```python
from build123d import *

# Parameters (mm, degrees)
FURO_COM_FOLGA_DE_M61_D = 6.4


with BuildPart() as part:
    # Esbo_o1 → Revolu_o1 (revolve)
    with BuildSketch(Plane(origin=(0, 0, 0), x_dir=(0, 0, -1), z_dir=(1, 0, 0)), mode=Mode.PRIVATE) as revolu_o1_sk:
        Polygon((-2, 6.5), (0, 6.5), (0, 0), (-7, 0), (-7, 6.5), (-4.7, 6.5), (-4.7, 4.3), (-2, 4.3), align=None)
    revolve(revolu_o1_sk.sketch.rotate(Axis((0, 0, 7), (0, 0, -1)), 90), axis=Axis((0, 0, 7), (0, 0, -1)))

    # Furo com folga de M61 (through all)
    with Locations(Plane(origin=(0, 0, 0), x_dir=(-1, 0, 0), z_dir=(0, 0, -1))):
        with Locations((0, 0)):
            Hole(FURO_COM_FOLGA_DE_M61_D / 2)


solid = part.part
```
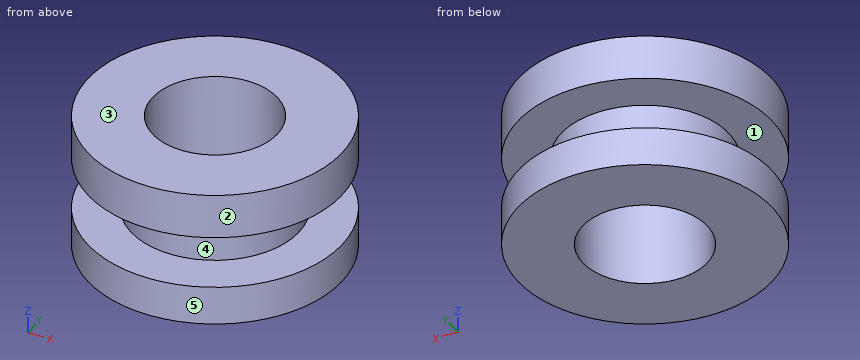
Input: part model. Units: mm. Frame: model coordinates. Face numbers are marked on the shaded views. A direction names the side the tool comes from. Round coordinates to 2 decimals unless told otherwise and drop trailing zeros. Loops run counter-clockwise (first coordinate to the right, second up) from the corner with the lowest first, then second, coordinate; pieces in that order, holes last. Notation, with made-up numbers: (30.5, 87.5) -> (44.5, 87.5) arc R18 ccw to (44.5, 111.5) -> close; hole circle Ø1 at (47, -30.75). An arc over 180 degrees is marked (long way). Use one line per item in the form item = value. Start each with the question number.
Item 1: Mould query, pull axis Z, two halves, no side actions, for the marked faces 3, 4 and 5. Classes: pulls with the +Z half, pulls with the -Z half, needs draft (parallel to the pull), parting line crosses it, or undercut.
Item 2: Section query C-C on z = 2.25. Return the cut outline in (x, y).
Item 3: Material intervals for L1, parallel to Y at x = 0, z = 4.75; L2, parallel to Y at x = 0, z = 2.5; L3, parallel to Z at x = 5.25, y = 2.5, sorted ascending. Write a range as from..to.
Item 4: Section query D-D on x = -4.5. Return the cut outline in (y, z).
Item 5: Set-up query: the marked faces 1 and 2. Return all of +Z, -Z, +X, -X, +Y, -Y with unobstructed straight access to the full face (end or side cutting, diameter ignored); none if empty.
Item 6: Contact query for flat-ended pins moving along their axis: pin 1 Ø4 at (x, z) = (4, 4) entering from -Y; pin 2 Ø4 at (y, z) = (-4, 2.5) entering from +X; pin 3 Ø1.5 at (x, z) = (3.5, 3.5) entering from +Y. Output: stop coordinate, or through.
Item 7: Section query A-A on y = 0. Return the cut outline in (x, z).
Ans:
q1.face_3 = pulls with the +Z half
q1.face_4 = undercut
q1.face_5 = needs draft
q2.outline = circle Ø8.6 at (0, 0); hole circle Ø6.4 at (0, 0)
q3.L1 = -6.5..-3.2, 3.2..6.5
q3.L2 = -4.3..-3.2, 3.2..4.3
q3.L3 = 0..2, 4.7..7
q4.outline = (-4.69, 0) -> (4.69, 0) -> (4.69, 2) -> (-4.69, 2) -> close; (-4.69, 4.7) -> (4.69, 4.7) -> (4.69, 7) -> (-4.69, 7) -> close
q5.face_1 = none
q5.face_2 = +Z, -Z
q6.pin_1 = -6.14
q6.pin_2 = 6.16
q6.pin_3 = 3.31
q7.outline = (-6.5, 0) -> (-3.2, 0) -> (-3.2, 7) -> (-6.5, 7) -> (-6.5, 4.7) -> (-4.3, 4.7) -> (-4.3, 2) -> (-6.5, 2) -> close; (3.2, 0) -> (6.5, 0) -> (6.5, 2) -> (4.3, 2) -> (4.3, 4.7) -> (6.5, 4.7) -> (6.5, 7) -> (3.2, 7) -> close
